The listing builds one solid part. Answer for the finished solid, in the listing's coordinates (mm). A direction names the side the tool comes from. Give positions to 0.01 mm unless a question says otherwise; leave off trailing zeros. Write each loop counter-clockwise with the first axis right and the second up, starting at its lowest first coordinate (ties: lowest second). Pieces come first, ordered by that corner, then holes.
```python
from build123d import *

# Parameters (mm, degrees)
SKETCH1_W           = 57
SKETCH1_H           = 21
BOSS_EXTRUDE1_DEPTH = 2.5
SKETCH2_W           = 42.5
SKETCH2_H           = 21
BOSS_EXTRUDE2_DEPTH = 5
SKETCH3_W           = 13
SKETCH3_H           = 3.5
CUT_EXTRUDE1_DEPTH  = 8.5


with BuildPart() as part:
    # Sketch1 → Boss-Extrude1 (new body)
    with BuildSketch(Plane.XY):
        Rectangle(SKETCH1_W, SKETCH1_H)
    extrude(amount=BOSS_EXTRUDE1_DEPTH)

    # Sketch2 → Boss-Extrude2 (add)
    with BuildSketch(Plane(origin=(0, 0, 0), x_dir=(-1, 0, 0), z_dir=(0, 0, -1))):
        Rectangle(SKETCH2_W, SKETCH2_H)
    extrude(amount=BOSS_EXTRUDE2_DEPTH)

    # Sketch3 → Cut-Extrude1 (cut, through all)
    with BuildSketch(Plane.XY.offset(2.5)):
        with Locations((0, 8.75)):
            Rectangle(SKETCH3_W, SKETCH3_H)
    cut_extrude1 = extrude(amount=-CUT_EXTRUDE1_DEPTH, mode=Mode.SUBTRACT)

    # Mirror1: Cut-Extrude1 across plane
    add(cut_extrude1.mirror(Plane.ZX), mode=Mode.SUBTRACT)


solid = part.part
```
Item 1: A cutting plane is placed at D-D, the plane y = -4.75. Give the vertices of the cut face in (x, z), plus the area to 3 significant figures.
Conclusion:
outline: (-28.5, 0) - (-21.25, 0) - (-21.25, -5) - (21.25, -5) - (21.25, 0) - (28.5, 0) - (28.5, 2.5) - (-28.5, 2.5) - close
area: 355 mm2
Item 2: Determine the mould class of faces 4 (the face through (21.25, 0, -2)), 5 (the face through (6.5, 9, -1)), 6 (the face through (-25, 0, 0)) for opening direction X: pulls with the +X half, pulls with the -X half, needs draft (parallel to the pull), parting line crosses it, or undercut.
Conclusion:
face 4: pulls with the +X half
face 5: undercut
face 6: needs draft
Item 3: Consider probe 1 along X at (y, z) = (-9.5, -2.5); probe 2 along Y at (x, z) = (0.5, 0.5); probe 3 along Z at (x, y) = (-24, -1.5). Determine where each line is inside the solid, lowest interval first.
Conclusion:
probe 1: x = -21.25 to -6.5, 6.5 to 21.25
probe 2: y = -7 to 7
probe 3: z = 0 to 2.5
Item 4: A cutting plane is placed at B-B, the plane z = 0.5. Give the vertices of the cut face in (x, y).
Conclusion:
outline: (-28.5, -10.5) - (-6.5, -10.5) - (-6.5, -7) - (6.5, -7) - (6.5, -10.5) - (28.5, -10.5) - (28.5, 10.5) - (6.5, 10.5) - (6.5, 7) - (-6.5, 7) - (-6.5, 10.5) - (-28.5, 10.5) - close
Item 5: Each of these flat-tipped pins is pushed along its axis until it touches: P1, Ø8, axis at x = 26, y = 3.5, coming from the -Z side; P2, Ø4, axis at x = -2, z = -2.5, coming from the -Y side; P3, Ø1.8, axis at y = -9.5, z = -2.5, coming from the +X side. Where does it stop, or does it pass through?
Conclusion:
P1: stops at z = 0
P2: stops at y = -7
P3: stops at x = 21.25
Item 6: Which of the six approach directions +Z, -Z, +X, -X, +Y, -Y give full straight-line access (tool end or side, diameter ignored) to faces 1 (the face through (-6.5, 9, -1)), 2 (the face through (6.5, -9, -1)), 3 (the face through (25, 0, 0))?
Conclusion:
face 1: +Z, -Z, +Y
face 2: +Z, -Z, -Y
face 3: -Z, +X, +Y, -Y
Item 7: A cutting plane is placed at C-C, the plane x = 1.5. Give the vertices of the cut face in (y, z).
Conclusion:
outline: (-7, -5) - (7, -5) - (7, 2.5) - (-7, 2.5) - close
Item 8: A cutting plane is placed at A-A, the plane y = 7.5. Give the vertices of the cut face in (x, z), plus the area to 4 significant figures.
Conclusion:
outline: (-28.5, 0) - (-21.25, 0) - (-21.25, -5) - (-6.5, -5) - (-6.5, 2.5) - (-28.5, 2.5) - close; (6.5, -5) - (21.25, -5) - (21.25, 0) - (28.5, 0) - (28.5, 2.5) - (6.5, 2.5) - close
area: 257.5 mm2
